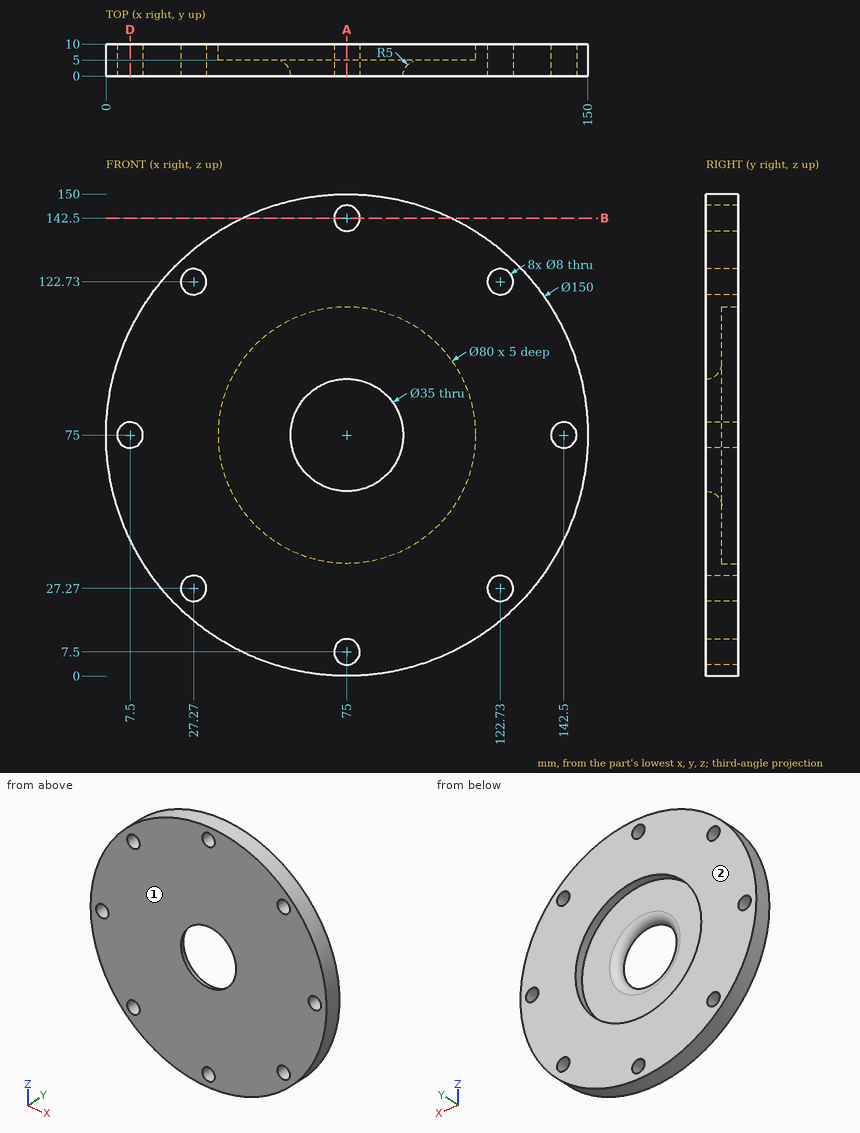
Can you work these out from the drawing? Everything is in mm from the part's minimum corner. Give positions to 0.01 mm unless a question says otherwise; leave off trailing zeros. Order: outer loops, then holes, each group sorted by start corner. A loop starts at its lowest first (then second) coordinate and runs counter-clockwise, first axis right, second up. Notation, with made-up numbers: M 41,50 L 60,50 A29 ccw 60,88 Z; hole C 39.25,-14 d5. An arc over 180 degrees is marked long. Use a Markdown table: item, result. Add a question column.
1. Suppose I cut it at B-B (z = 142.5). List the corners of the cut face in (x, y) for me.
2. I need wall thicknesses on probe 1 along Z at (x, y) = (78, 3) (1 decimal); probe 2 along Y at (x, z) = (40.5, 55); probe 3 along X at (y, z) = (9.75, 74). Which ranges of each line are inside material? Lowest first, please. Write a range as from..to.
3. Suppose I cut it at D-D (x = 7.5). List the corners of the cut face in (y, z) for me.
4. Suppose I cut it at A-A (x = 75). Give the number of separate pieces and of enclosed holes in the cut face.
5. For pin 1 Ø4 at (x, y) = (64.5, 4.5) entering from -Z; pin 2 Ø21 at (x, z) = (75, 75) entering from +Y; pin 3 Ø2 at (x, y) = (79, 8.5) entering from +Z; pin 4 Ø1.5 at (y, z) = (9, 67.5) entering from +X (1 decimal), each with a flat end and sliding along its axis, tell me the tip position at first contact or that it passes through.
6. If we mould it in two halves opening along Y, with no side actions, what happens to the marked faces 1 and 2? For each: +Y half, -Y half, draft (parallel to the pull), parting line (faces both ways), or undercut.
Results list:
| question | item | result |
|---|---|---|
| 1 | outline | M 42.31,0 L 71,0 L 71,10 L 42.31,10 Z; M 79,0 L 107.69,0 L 107.69,10 L 79,10 Z |
| 2 | probe 1 | z = 0.1..4.9, 10.1..56.7, 93.3..139.9, 145.1..149.9 |
| 2 | probe 2 | y = 0..5 |
| 2 | probe 3 | x = 0.01..3.63, 11.37..35.01, 114.99..138.63, 146.37..149.99 |
| 3 | outline | M 0,42.31 L 10,42.31 L 10,71 L 0,71 Z; M 0,79 L 10,79 L 10,107.69 L 0,107.69 Z |
| 4 | separate pieces | 4 |
| 4 | enclosed holes | 0 |
| 5 | pin 1 | stops at z = 0.48 |
| 5 | pin 2 | passes through |
| 5 | pin 3 | stops at z = 149.94 |
| 5 | pin 4 | stops at x = 149.7 |
| 6 | face 1 | -Y half |
| 6 | face 2 | +Y half |
